Can you work these out from the model? Positions are in its coordinate system, mm. Coordinates: 2 decimals unless noted, no trailing zeros. Order: outer loops, then holes, each group sorted by start corner. A loop starts at its lowest first (then second) coordinate and runs counter-clockwise, first axis right, second up. Notation, with made-up numbers: M 71,18.5 L 125,18.5 A20 ccw 125,38.5 Z; hole C 84.5,23.5 d11. An arc over 180 degrees is marked long. Answer as a JSON object with one key per item and string values.
from build123d import *

# Parameters (mm, degrees)
CROQUIS1_W              = 80
CROQUIS1_H              = 65
SALIENTE_EXTRUIR1_DEPTH = 2.5
CORTAR_EXTRUIR1_REACH   = 53.599
CROQUIS2_R              = 2
REDONDEO1_R             = 2.5
CHAFL_N1_SIZE           = 1


with BuildPart() as part:
    # Croquis1 → Saliente-Extruir1 (new body)
    with BuildSketch(Plane(origin=(0, 0, 0), x_dir=(1, 0, 0), z_dir=(0, 1, 0))):
        Rectangle(CROQUIS1_W, CROQUIS1_H)
    extrude(amount=SALIENTE_EXTRUIR1_DEPTH)

    # Croquis2 → Cortar-Extruir1 (cut, up to next)
    with BuildSketch(Plane(origin=(0, 2.5, 0), x_dir=(1, 0, 0), z_dir=(0, 1, 0)), mode=Mode.PRIVATE) as cortar_extruir1_sk1:
        with Locations(Location((-36, 28.5, 0), (0, 0, 270))):
            Circle(CROQUIS2_R)
    cortar_extruir1_tool1 = extrude(cortar_extruir1_sk1.sketch, amount=-CORTAR_EXTRUIR1_REACH, mode=Mode.PRIVATE) & part.part
    # Croquis2 → Cortar-Extruir1 (cut, up to next)
    with BuildSketch(Plane(origin=(0, 2.5, 0), x_dir=(1, 0, 0), z_dir=(0, 1, 0)), mode=Mode.PRIVATE) as cortar_extruir1_sk2:
        with Locations(Location((36, 28.5, 0), (0, 0, 270))):
            Circle(CROQUIS2_R)
    cortar_extruir1_tool2 = extrude(cortar_extruir1_sk2.sketch, amount=-CORTAR_EXTRUIR1_REACH, mode=Mode.PRIVATE) & part.part
    # Croquis2 → Cortar-Extruir1 (cut, up to next)
    with BuildSketch(Plane(origin=(0, 2.5, 0), x_dir=(1, 0, 0), z_dir=(0, 1, 0)), mode=Mode.PRIVATE) as cortar_extruir1_sk3:
        with Locations(Location((-36, -28.5, 0), (0, 0, 270))):
            Circle(CROQUIS2_R)
    cortar_extruir1_tool3 = extrude(cortar_extruir1_sk3.sketch, amount=-CORTAR_EXTRUIR1_REACH, mode=Mode.PRIVATE) & part.part
    # Croquis2 → Cortar-Extruir1 (cut, up to next)
    with BuildSketch(Plane(origin=(0, 2.5, 0), x_dir=(1, 0, 0), z_dir=(0, 1, 0)), mode=Mode.PRIVATE) as cortar_extruir1_sk4:
        with Locations(Location((36, -28.5, 0), (0, 0, 270))):
            Circle(CROQUIS2_R)
    cortar_extruir1_tool4 = extrude(cortar_extruir1_sk4.sketch, amount=-CORTAR_EXTRUIR1_REACH, mode=Mode.PRIVATE) & part.part
    add(cortar_extruir1_tool1.solids().sort_by_distance((-36, 2.5, -28.5))[0], mode=Mode.SUBTRACT)
    add(cortar_extruir1_tool2.solids().sort_by_distance((36, 2.5, -28.5))[0], mode=Mode.SUBTRACT)
    add(cortar_extruir1_tool3.solids().sort_by_distance((-36, 2.5, 28.5))[0], mode=Mode.SUBTRACT)
    add(cortar_extruir1_tool4.solids().sort_by_distance((36, 2.5, 28.5))[0], mode=Mode.SUBTRACT)

    # Redondeo1
    redondeo1_edges = [part.edges().sort_by_distance(p)[0] for p in [
        (-40, 1.25, -32.5),
        (40, 1.25, -32.5),
        (40, 1.25, 32.5),
        (-40, 1.25, 32.5),
    ]]
    fillet(redondeo1_edges, radius=REDONDEO1_R)

    # Chaflán1
    chafl_n1_edges = [part.edges().sort_by_distance(p)[0] for p in [
        (36, 2.5, -30.5),
        (-36, 2.5, 26.5),
        (36, 2.5, 26.5),
        (-36, 2.5, -30.5),
    ]]
    chamfer(chafl_n1_edges, length=CHAFL_N1_SIZE)


solid = part.part
Item 1: I want a section at B-B, the plane z = -28.5. Write out the boundary of the cut face in (x, y).
Answers follow:
{"outline": "M -40,0 L -38,0 L -38,1.5 L -39,2.5 L -40,2.5 Z; M -34,0 L 34,0 L 34,1.5 L 33,2.5 L -33,2.5 L -34,1.5 Z; M 38,0 L 40,0 L 40,2.5 L 39,2.5 L 38,1.5 Z"}
Item 2: I want a section at C-C, the plane y = 2.1. Write out the boundary of the cut face in (x, z).
Answers follow:
{"outline": "M -40,-30 A2.5 ccw -37.5,-32.5 L 37.5,-32.5 A2.5 ccw 40,-30 L 40,30 A2.5 ccw 37.5,32.5 L -37.5,32.5 A2.5 ccw -40,30 Z; hole C -36,-28.5 d5.2; hole C -36,28.5 d5.2; hole C 36,-28.5 d5.2; hole C 36,28.5 d5.2"}
Item 3: I want a section at A-A, the plane x = 36. Write out the boundary of the cut face in (y, z).
Answers follow:
{"outline": "M 0,-32.5 L 2.5,-32.5 L 2.5,-31.5 L 1.5,-30.5 L 0,-30.5 Z; M 0,-26.5 L 1.5,-26.5 L 2.5,-25.5 L 2.5,25.5 L 1.5,26.5 L 0,26.5 Z; M 0,30.5 L 1.5,30.5 L 2.5,31.5 L 2.5,32.5 L 0,32.5 Z"}
Item 4: If we mould it in two halves opening along Z, with no side actions, what happens to faces 1 (the cylindrical face through (34.226, 0.76, -27.577)), 2 (the flat face through (-1, 1, 32.5)), 3 (the cylindrical face through (39, 1, -32))? For each: pulls with the +Z half, pulls with the -Z half, needs draft (parallel to the pull), parting line crosses it, or undercut.
Answers follow:
{"face 1": "undercut", "face 2": "pulls with the +Z half", "face 3": "pulls with the -Z half"}
Item 5: Please list where these lines run through material, in increasing order: line 1 (X direction, y = 2.1, z = 28); line 2 (X direction, y = 1.15, z = 27.5).
Answers follow:
{"line 1": "x = -40 to -38.55, -33.45 to 33.45, 38.55 to 40", "line 2": "x = -40 to -37.73, -34.27 to 34.27, 37.73 to 40"}
